Part model, mm, in its own coordinate system. Give positions to 0.01 mm unless a question says otherwise; leave off trailing zeros. Order: outer loops, then holes, each group sorted by start corner. A loop starts at its lowest first (then second) coordinate and runs counter-clockwise, first axis right, second up. Notation, with made-up numbers: (61, -9.5) - (89, -9.5) arc R17 ccw to (89, 6.5) - close; hole circle Ø11 at (-11, 45). An arc over 180 degrees is marked (long way). One line per item, written item: value.
```python
from build123d import *

# Parameters (mm, degrees)
BOSS_EXTRUDE1_DEPTH = 3
CUT_EXTRUDE1_REACH  = 5
SKETCH2_R           = 2
CUT_EXTRUDE2_REACH  = 5
SKETCH3_R           = 2
SKETCH4_W           = 10
SKETCH4_H           = 3
BOSS_EXTRUDE3_DEPTH = 2.7
SKETCH5_W           = 10
SKETCH5_H           = 3
BOSS_EXTRUDE4_DEPTH = 2.7
CUT_EXTRUDE3_REACH  = 5
SKETCH6_W           = 13
SKETCH6_H           = 5


with BuildPart() as part:
    # Sketch1 → Boss-Extrude1 (new body)
    with BuildSketch(Plane(origin=(0, 0, 0), x_dir=(1, 0, 0), z_dir=(0, 1, 0))):
        Polygon((101.124303582, 11.213732055), (101.124303582, 66.273277114), (40.502525317, 31.273277114), (-168.875696418, 31.273277114), (-168.875696418, -18.726722886), (101.124303582, -18.726722886), align=None)
    extrude(amount=BOSS_EXTRUDE1_DEPTH)

    # Sketch2 → Cut-Extrude1 (cut, up to next)
    with BuildSketch(Plane(origin=(0, 3, 0), x_dir=(1, 0, 0), z_dir=(0, 1, 0)), mode=Mode.PRIVATE) as cut_extrude1_sk1:
        with Locations(Location((-152.875696418, 6.273277114, 0), (0, 0, 270))):  # turned: the seam where the file's is
            Circle(SKETCH2_R)
    cut_extrude1_tool1 = extrude(cut_extrude1_sk1.sketch, amount=-CUT_EXTRUDE1_REACH, mode=Mode.PRIVATE) & part.part
    add(cut_extrude1_tool1.solids().sort_by_distance((-152.875696, 3, -6.273277))[0], mode=Mode.SUBTRACT)
    # Sketch2 → Cut-Extrude1 (cut, up to next)
    with BuildSketch(Plane(origin=(0, 3, 0), x_dir=(1, 0, 0), z_dir=(0, 1, 0)), mode=Mode.PRIVATE) as cut_extrude1_sk2:
        with Locations(Location((85.124303582, 23.773277114, 0), (0, 0, 270))):  # turned: the seam where the file's is
            Circle(SKETCH2_R)
    cut_extrude1_tool2 = extrude(cut_extrude1_sk2.sketch, amount=-CUT_EXTRUDE1_REACH, mode=Mode.PRIVATE) & part.part
    add(cut_extrude1_tool2.solids().sort_by_distance((85.124304, 3, -23.773277))[0], mode=Mode.SUBTRACT)

    # Sketch3 → Cut-Extrude2 (cut, up to next)
    with BuildSketch(Plane(origin=(0, 3, 0), x_dir=(1, 0, 0), z_dir=(0, 1, 0)), mode=Mode.PRIVATE) as cut_extrude2_sk1:
        with Locations(Location((-128.875696418, -2.726722886, 0), (0, 0, 270))):  # turned: the seam where the file's is
            Circle(SKETCH3_R)
    cut_extrude2_tool1 = extrude(cut_extrude2_sk1.sketch, amount=-CUT_EXTRUDE2_REACH, mode=Mode.PRIVATE) & part.part
    add(cut_extrude2_tool1.solids().sort_by_distance((-128.875696, 3, 2.726723))[0], mode=Mode.SUBTRACT)
    # Sketch3 → Cut-Extrude2 (cut, up to next)
    with BuildSketch(Plane(origin=(0, 3, 0), x_dir=(1, 0, 0), z_dir=(0, 1, 0)), mode=Mode.PRIVATE) as cut_extrude2_sk2:
        with Locations(Location((61.124303582, -2.726722886, 0), (0, 0, 270))):  # turned: the seam where the file's is
            Circle(SKETCH3_R)
    cut_extrude2_tool2 = extrude(cut_extrude2_sk2.sketch, amount=-CUT_EXTRUDE2_REACH, mode=Mode.PRIVATE) & part.part
    add(cut_extrude2_tool2.solids().sort_by_distance((61.124304, 3, 2.726723))[0], mode=Mode.SUBTRACT)

    # Sketch4 → Boss-Extrude3 (add)
    with BuildSketch(Plane.XY.offset(-31.273277114)):
        with Locations((-148.875696418, 1.5)):
            Rectangle(SKETCH4_W, SKETCH4_H)
        with Locations((20.502525317, 1.5)):
            Rectangle(SKETCH4_W, SKETCH4_H)
    extrude(amount=-BOSS_EXTRUDE3_DEPTH)

    # Sketch5 → Boss-Extrude4 (add)
    with BuildSketch(Plane(origin=(-3.416094891, 0, -5.916849915), x_dir=(-0.866025404, 0, 0.5), z_dir=(-0.5, 0, -0.866025404))):
        with Locations((-85.712854399, 1.5)):
            Rectangle(SKETCH5_W, SKETCH5_H)
    extrude(amount=BOSS_EXTRUDE4_DEPTH)

    # Sketch6 → Cut-Extrude3 (cut, up to next)
    with BuildSketch(Plane(origin=(0, 3, 0), x_dir=(1, 0, 0), z_dir=(0, 1, 0)), mode=Mode.PRIVATE) as cut_extrude3_sk1:
        with Locations((-108.875696418, -6.726722886)):
            Rectangle(SKETCH6_W, SKETCH6_H)
    cut_extrude3_tool1 = extrude(cut_extrude3_sk1.sketch, amount=-CUT_EXTRUDE3_REACH, mode=Mode.PRIVATE) & part.part
    add(cut_extrude3_tool1.solids().sort_by_distance((-108.875696, 3, 6.726723))[0], mode=Mode.SUBTRACT)


solid = part.part
```
1) Cut at A-A, the plane x = -111. Give the cut face in (y, z), then the cut area to 3 significant figures.
Outcome:
outline: (0, -31.27) - (3, -31.27) - (3, 4.23) - (0, 4.23) - close; (0, 9.23) - (3, 9.23) - (3, 18.73) - (0, 18.73) - close
area: 135 mm^2
2) Cut at C-C, the plane x = -42. Give the cut face in (y, z), then the cut area to 3 significant figures.
Outcome:
outline: (0, -31.27) - (3, -31.27) - (3, 18.73) - (0, 18.73) - close
area: 150 mm^2
3) Drill centre lines: line 1 along Z through (x, y) = (-129, 0.2); line 2 along Z through (x, y) = (-111, 2.4); line 3 along X through (y, z) = (0.5, -23.5). Where is each one in solid material? Low to high. Write a range as from..to.
Outcome:
line 1: z = -31.27..0.73, 4.72..18.73
line 2: z = -31.27..4.23, 9.23..18.73
line 3: x = -168.88..83.14, 87.11..101.12
4) Pin check, flat tips, straight feed: pin 1 (0.9 mm diameter, centred on x = -148, y = 2, fed in from -Z); pin 2 (1.3 mm diameter, centred on y = 1, z = -33, fed in from -X); pin 3 (0.9 mm diameter, centred on x = -164, y = 1.5, fed in from -Z); pin 4 (3.5 mm diameter, centred on x = 85.12, z = -23.77, fed in from +Y). Stop position of each tip, or through.
Outcome:
pin 1: stops at z = -33.97
pin 2: stops at x = -153.88
pin 3: stops at z = -31.27
pin 4: passes through
5) Cut at B-B, the plane y = 1.5. Give the cut face in (x, z).
Outcome:
outline: (-168.88, -31.27) - (-153.88, -31.27) - (-153.88, -33.97) - (-143.88, -33.97) - (-143.88, -31.27) - (15.5, -31.27) - (15.5, -33.97) - (25.5, -33.97) - (25.5, -31.27) - (40.5, -31.27) - (66.48, -46.27) - (65.13, -48.61) - (73.79, -53.61) - (75.14, -51.27) - (101.12, -66.27) - (101.12, 18.73) - (-168.88, 18.73) - close; hole circle Ø4 at (-152.88, -6.27); hole circle Ø4 at (-128.88, 2.73); hole (-115.38, 4.23) - (-102.38, 4.23) - (-102.38, 9.23) - (-115.38, 9.23) - close; hole circle Ø4 at (61.12, 2.73); hole circle Ø4 at (85.12, -23.77)
